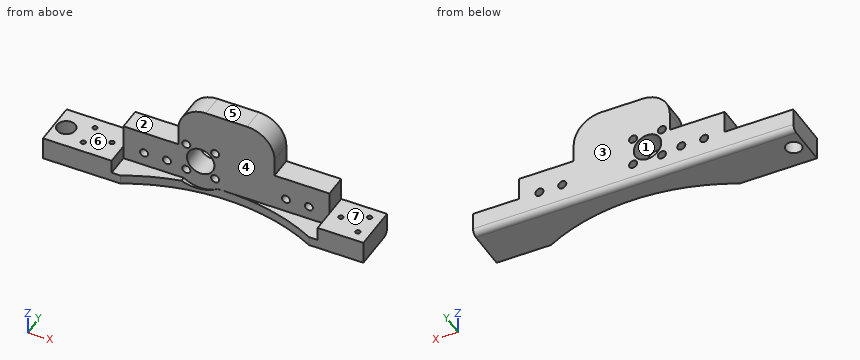
Autodesk Inventor part; units mm, degrees
ref_plane "YZ Plane" through (0, 0, 0) normal (1, 0, 0) x (0, 1, 0)
ref_plane "XZ Plane" through (0, 0, 0) normal (0, 1, 0) x (-1, 0, 0)
ref_plane "XY Plane" through (0, 0, 0) normal (0, 0, 1) x (1, 0, 0)
sketch "Sketch1" plane through (0, 0, 0) normal (1, 0, 0) x (0, 1, 0)
  line L0 (11.2985, 26.2091) -> (-1.4015, 26.2091)
  line L1 (-1.4015, 26.2091) -> (-1.4015, -24.5909)
  line L2 (-1.4015, -24.5909) -> (11.2985, -24.5909)
  line L3 (11.2985, -24.5909) -> (11.2985, 26.2091)
  point P0 (0, 0)
  dimension "d0" = 50.8
  dimension "d1" = 12.7
extrude "Extrusion1" add sketch "Sketch1" along normal blind 165.1
sketch "Sketch2" plane through (0, 11.2985, 26.2091) normal (0, 1, 0) x (1, 0, 0)
  circle A0 centre (68.2625, 31.75) radius 12.7
  circle A1 centre (87.3125, 31.75) radius 12.7
  line L0 (0, 50.8) -> (0, 0)
  line L1 (0, 50.8) -> (165.1, 50.8)
  point P0 (0, 26.2091)
  point P1 (60.2615, 39.751)
  point P2 (76.2635, 39.751)
  point P3 (76.2635, 23.749)
  point P4 (60.2615, 23.749)
  dimension "d4" = 25.4
  dimension "d5" = 25.4
  dimension "d6" = 0
  dimension "d7" = 19.05
  dimension "d8" = 68.2625
  dimension "d9" = 19.05
  dimension "d46" = 0
  dimension "d47" = 0
  dimension "d48" = 0
  dimension "d49" = 0
  dimension "d50" = 16.002
  dimension "d51" = 16.002
  dimension "d52" = 8.001
  dimension "d53" = 8.001
sketch "Sketch8" plane through (0, 11.2985, 26.2091) normal (0, 1, 0) x (1, 0, 0)
  line L0 (-37.599, -14.8006) -> (55.88, -14.8006)
  line L1 (55.88, -14.8006) -> (55.88, 38.1)
  line L2 (55.88, 38.1) -> (-37.599, 38.1)
  line L3 (-37.599, 38.1) -> (-37.599, -14.8006)
  line L4 (109.22, -16.386) -> (193.9952, -16.386)
  line L5 (193.9952, -16.386) -> (193.9952, 38.1)
  line L6 (193.9952, 38.1) -> (109.22, 38.1)
  line L7 (109.22, 38.1) -> (109.22, -16.386)
  line L8 (0, 50.8) -> (165.1, 50.8)
  line L9 (0, 50.8) -> (0, 0)
  line L10 (165.1, 50.8) -> (165.1, 0)
  point P0 (0, 26.2091)
  dimension "d36" = 12.7
  dimension "d37" = 55.88
  dimension "d38" = 12.7
  dimension "d39" = 55.88
extrude "Extrusion8" cut sketch "Sketch8" against normal blind 76.2
fillet "Fillet1" radius 15.24 1 edges at (109.22, 4.9485, 26.2091)
fillet "Fillet2" radius 15.24 1 edges at (55.88, 4.9485, 26.2091)
hole "Hole1" at (60.2615, 11.2985, -13.5419) at (76.2635, 11.2985, -13.5419) at (76.2635, 11.2985, 2.4601) at (60.2615, 11.2985, 2.4601) direction (0, -1, 0) diameter 4.4958 end through all
sketch "Sketch10" plane through (0, 11.2985, -24.5909) normal (0, 1, 0) x (1, 0, 0)
  circle A0 centre (76.2635, -27.051) radius 2.2479
  circle A1 centre (60.2615, -11.049) radius 2.2479
  circle A2 centre (60.2615, -27.051) radius 2.2479
  circle A3 centre (76.2635, -11.049) radius 2.2479
  line L0 (76.2635, -11.049) -> (60.2615, -27.051)
  line L1 (60.2615, -11.049) -> (76.2635, -27.051)
  point P0 (0, -24.5909)
  point P1 (68.2625, -19.05)
  dimension "d61" = 8.001
  dimension "d62" = 8.001
hole "Hole2" at (68.2625, 11.2985, -5.5409) direction (0, -1, 0) diameter 15.24 end through all
sketch "Sketch11" plane through (0, 11.2985, -11.8909) normal (0, 0, 1) x (1, 0, 0)
  line L0 (55.88, 0) -> (0, 0)
  line L1 (0, 0) -> (0, -12.7)
  line L2 (0, -12.7) -> (55.88, -12.7)
  line L3 (55.88, -12.7) -> (55.88, 0)
  line L4 (0, -12.7) -> (0, 0)
  line L5 (55.88, 0) -> (55.88, -12.7)
  line L6 (0, 0) -> (55.88, 0)
  line L7 (55.88, -12.7) -> (0, -12.7)
  point P0 (0, -11.2985)
  dimension "d70" = 0
  dimension "d71" = 0
  dimension "d72" = 0
  dimension "d73" = 0
extrude "Extrusion9" add sketch "Sketch11" along normal blind 12.7
sketch "Sketch12" plane through (109.22, 11.2985, -11.8909) normal (0, 0, 1) x (1, 0, 0)
  line L0 (0, 0) -> (55.88, 0)
  line L1 (55.88, 0) -> (55.88, -12.7)
  line L2 (55.88, -12.7) -> (0, -12.7)
  line L3 (0, -12.7) -> (0, 0)
  line L4 (55.88, 0) -> (55.88, -12.7)
  line L5 (0, 0) -> (55.88, 0)
  line L6 (55.88, -12.7) -> (0, -12.7)
  line L7 (0, -12.7) -> (0, 0)
  point P0 (-109.22, -11.2985)
  dimension "d76" = 0
  dimension "d77" = 0
  dimension "d78" = 0
  dimension "d79" = 0
extrude "Extrusion10" add sketch "Sketch12" along normal blind 12.7
sketch "Sketch13" plane through (0, 11.2985, -24.5909) normal (0, 1, 0) x (1, 0, 0)
  line L0 (55.88, -25.4) -> (55.88, -35.56)
  line L1 (0, 0) -> (165.1, 0)
  line L2 (109.22, -35.56) -> (109.22, -25.4)
  point P0 (0, -24.5909)
  point P1 (49.53, -12.7)
  point P2 (36.83, -12.7)
  point P3 (115.57, -12.7)
  point P4 (128.27, -12.7)
  dimension "d82" = 19.05
  dimension "d83" = 6.35
  dimension "d84" = 12.7
  dimension "d85" = 12.7
  dimension "d86" = 6.35
  dimension "d87" = 19.05
  dimension "d88" = 12.7
  dimension "d89" = 12.7
hole "Hole3" at (49.53, 11.2985, -11.8909) at (36.83, 11.2985, -11.8909) at (115.57, 11.2985, -11.8909) at (128.27, 11.2985, -11.8909) direction (0, -1, 0) diameter 4.4958 depth 25.4 tip angle 118.188
sketch "Sketch14" plane through (0, 11.2985, -24.5909) normal (0, 1, 0) x (1, 0, 0)
  line L0 (0, 0) -> (25.4, 0)
  line L1 (25.4, 0) -> (25.4, -25.4)
  line L2 (25.4, -25.4) -> (0, -25.4)
  line L3 (0, -25.4) -> (0, 0)
  line L4 (165.1, 0) -> (139.7, 0)
  line L5 (139.7, 0) -> (139.7, -25.4)
  line L6 (139.7, -25.4) -> (165.1, -25.4)
  line L7 (165.1, -25.4) -> (165.1, 0)
  line L8 (0, 0) -> (165.1, 0)
  line L9 (165.1, 0) -> (165.1, -25.4)
  line L10 (165.1, -25.4) -> (109.22, -25.4)
  line L11 (0, 0) -> (0, -25.4)
  line L12 (55.88, -25.4) -> (0, -25.4)
  point P0 (0, -24.5909)
  dimension "d97" = 0
  dimension "d98" = 25.4
  dimension "d99" = 0
  dimension "d100" = 0
  dimension "d101" = 25.4
  dimension "d102" = 0
  dimension "d103" = 0
  dimension "d104" = 0
extrude "Extrusion11" add sketch "Sketch14" against normal blind 25.4
sketch "Sketch16" plane through (0, -14.1015, -24.5909) normal (0, -1, 0) x (1, 0, 0)
  line L0 (-15.071, 42.5671) -> (25.4, 42.5671)
  line L1 (25.4, 42.5671) -> (25.4, 12.7)
  line L2 (25.4, 12.7) -> (-15.071, 12.7)
  line L3 (-15.071, 12.7) -> (-15.071, 42.5671)
  line L4 (139.7, 42.5671) -> (181.0335, 42.5671)
  line L5 (181.0335, 42.5671) -> (181.0335, 12.7)
  line L6 (181.0335, 12.7) -> (139.7, 12.7)
  line L7 (139.7, 12.7) -> (139.7, 42.5671)
  line L8 (165.1, 25.4) -> (139.7, 25.4)
  line L9 (139.7, 25.4) -> (139.7, 0)
  line L10 (25.4, 0) -> (25.4, 25.4)
  line L11 (25.4, 25.4) -> (0, 25.4)
  point P0 (0, 24.5909)
  dimension "d112" = 12.7
  dimension "d113" = 0
  dimension "d114" = 0
  dimension "d115" = 12.7
extrude "Extrusion13" cut sketch "Sketch16" against normal blind 50.8
sketch "Sketch17" plane through (0, -14.1015, -11.8909) normal (0, 0, 1) x (1, 0, 0)
  line L0 (0, 0) -> (0, 25.4)
  line L1 (0, 25.4) -> (25.4, 25.4)
  line L2 (25.4, 0) -> (0, 0)
  line L3 (165.1, 25.4) -> (165.1, 0)
  line L4 (139.7, 25.4) -> (165.1, 25.4)
  line L5 (165.1, 0) -> (139.7, 0)
  point P0 (0, 14.1015)
  point P1 (6.35, 19.05)
  point P2 (6.35, 6.35)
  point P3 (19.05, 12.7)
  point P4 (146.05, 12.7)
  point P5 (158.75, 19.05)
  point P6 (158.75, 6.35)
  dimension "d118" = 6.35
  dimension "d119" = 6.35
  dimension "d120" = 6.35
  dimension "d121" = 6.35
  dimension "d122" = 19.05
  dimension "d123" = 12.7
  dimension "d124" = 19.05
  dimension "d125" = 12.7
  dimension "d126" = 6.35
  dimension "d127" = 6.35
  dimension "d128" = 6.35
  dimension "d129" = 6.35
hole "Hole4" at (6.35, 4.9485, -11.8909) at (6.35, -7.7515, -11.8909) at (19.05, -1.4015, -11.8909) at (146.05, -1.4015, -11.8909) at (158.75, 4.9485, -11.8909) at (158.75, -7.7515, -11.8909) direction (0, 0, -1) diameter 2.6416 depth 10.9728 tip angle 118.188
sketch "Sketch18" plane through (71.12, -1.4015, 26.2091) normal (0, -1, 0) x (1, 0, 0)
  line L0 (-45.72, -45.72) -> (68.58, -45.72)
  line L1 (68.58, -45.72) -> (68.58, -50.8)
  line L2 (68.58, -50.8) -> (-45.72, -50.8)
  line L3 (-45.72, -50.8) -> (-45.72, -45.72)
  line L4 (-45.72, -50.8) -> (68.58, -50.8)
  line L5 (68.58, -38.1) -> (68.58, -50.8)
  line L6 (-45.72, -50.8) -> (-45.72, -38.1)
  point P0 (-71.12, -26.2091)
  dimension "d137" = 0
  dimension "d138" = 0
  dimension "d139" = 5.08
  dimension "d140" = 0
extrude "Extrusion14" add sketch "Sketch18" along normal blind 12.7
sketch "Sketch19" plane through (165.1, 11.2985, -24.5909) normal (0, 0, -1) x (-1, 0, 0)
  line L0 (82.55, -51.592) -> (82.55, 23.9487)
  line L1 (165.1, 0) -> (165.1, -25.4)
  line L2 (0, 0) -> (0, -25.4)
  arc A0 (134.9134, -25.4) -> (30.1866, -25.4) centre (82.55, -127) ccw
  line L3 (165.1, -25.4) -> (0, -25.4)
  line L4 (134.9134, -25.4) -> (30.1866, -25.4)
  point P0 (165.1, -11.2985)
  dimension "d143" = 82.55
  dimension "d144" = 82.55
  dimension "d145" = 0
  dimension "d146" = 101.6
  dimension "d147" = 228.6
extrude "Extrusion15" cut sketch "Sketch19" against normal blind 6.35
sketch "Sketch20" plane through (0, 0, 0) normal (-1, 0, 0) x (0, 0, 1)
  line L0 (-24.5909, 11.2985) -> (-24.5909, -14.1015)
  line L1 (-11.8909, -14.1015) -> (-24.5909, -14.1015)
  line L2 (-11.8909, -14.1015) -> (-11.8909, 11.2985)
  line L3 (-24.5909, 11.2985) -> (-11.8909, 11.2985)
  line L4 (-11.8909, -14.1015) -> (-11.8909, -1.4015)
  line L5 (-11.8909, -14.1015) -> (-24.5909, -14.1015)
  line L6 (-24.5909, -14.1015) -> (-24.5909, 11.2985)
  line L7 (-24.5909, 11.2985) -> (-11.8909, 11.2985)
  line L8 (-11.8909, 11.2985) -> (-11.8909, -14.1015)
  point P0 (0, 0)
extrude "Extrusion16" add sketch "Sketch20" along normal blind 12.7
sketch "Sketch21" plane through (25.4, -14.1015, -11.8909) normal (0, 0, 1) x (1, 0, 0)
  line L0 (0, 0) -> (-38.1, 0)
  line L1 (-38.1, 0) -> (-38.1, 25.4)
  point P0 (-25.4, 14.1015)
  point P1 (-31.75, 12.7)
  dimension "d152" = 12.7
  dimension "d153" = 6.35
hole "Hole5" at (-6.35, -1.4015, -11.8909) direction (0, 0, -1) diameter 10.16 depth 12.2936 tip angle 118.188
fillet "Fillet3" radius 3.175 1 edges at (76.2, 11.2985, -24.5909)
sketch "Sketch22" plane through (71.12, -1.4015, 26.2091) normal (0, -1, 0) x (1, 0, 0)
  circle A0 centre (-2.8575, -31.75) radius 7.62
  circle A1 centre (-2.8575, -31.75) radius 16.8231
  point P0 (-71.12, -26.2091)
extrude "Extrusion17" cut sketch "Sketch22" along normal blind 25.4
properties part number "GripperM otorBlock"
Check sheet for the modelled part. Datum: model origin and axes. Units: mm. Face numbers are marked on the shaded views. A direction names the side the tool comes from. Round coordinates to 2 decimals unless told otherwise and drop trailing zeros. Loops run counter-clockwise (first coordinate to the right, second up) from the corner with the lowest first, then second, coordinate; pieces in that order, holes last. Notation, with made-up numbers: (53.5, 54.5) - (68.5, 54.5) arc R9 cw to (68.5, 58.5) - close; hole circle Ø1 at (-21.5, 58.5). An arc over 180 degrees is marked (long way). Write item = value, one per line. Start each with the question number.
Q1. Release check for a two-part mould opening along Z. For the marked faces 1, 2 and 3 record: pulls with the +Z half, pulls with the -Z half, needs draft (parallel to the pull), parting line crosses it, or undercut.
Q2. Section check D-D (z = 9). Record the boundary of the cut face in (x, y), plus the area to 3 significant figures.
Q3. Section check B-B (z = -7). Record the boundary of the cut face in (x, y).
Q4. Depth check by flat-ended pin: P1, Ø4, axis at y = 4.5, z = -4, coming from the +X side; P2, Ø8, axis at x = -6.35, y = -1.4, coming from the +Z side; P3, Ø6, axis at y = -5.5, z = -10, coming from the -X side; P4, Ø10, axis at x = 38, y = 8, coming from the +Z side. Enter the tip coordinate at first touch or a pass-through.
Q5. Access from +Z, -Z, +X, -X, +Y, -Y to the whole of each face (thin tool, end or side, straight path). Record for the marked faces 4, 5, 6 and 7.
Q6. Thickness scan on L1, parallel to Y at x = 6.35, z = -15; L2, parallel to Z at x = 115.57, y = 8; L3, parallel to Y at x = 19.05, z = -17.75. Record the ranges inside material, lowest first.
Derived:
q1.face_1 = undercut
q1.face_2 = pulls with the +Z half
q1.face_3 = needs draft
q2.outline = (55.88, -1.4) - (109.22, -1.4) - (109.22, 11.3) - (55.88, 11.3) - close
q2.area = 677 mm^2
q3.outline = (25.4, -1.4) - (60.78, -1.4) - (60.78, 11.3) - (25.4, 11.3) - close; (75.74, -1.4) - (139.7, -1.4) - (139.7, 11.3) - (75.74, 11.3) - close
q4.P1 = 139.7
q4.P2 = through
q4.P3 = -12.7
q4.P4 = 0.81
q5.face_4 = +Z, -Y
q5.face_5 = +Z, +X, -X, +Y, -Y
q5.face_6 = +Z, -X, +Y, -Y
q5.face_7 = +Z, +X, +Y, -Y
q6.L1 = -14.1 to -9.07, -6.43 to 3.63, 6.27 to 11.3
q6.L2 = -24.59 to -14.14, -9.64 to 0.81
q6.L3 = -14.1 to -2.72, -0.08 to 11.3
